Part model, mm, in its own coordinate system. A direction names the side the tool comes from. Round coordinates to 2 decimals unless told otherwise and drop trailing zeros. Write each loop counter-clockwise with the first axis right and the second up, starting at its lowest first coordinate (ties: lowest second). Pieces come first, ordered by that corner, then holes. Notation, with made-up numbers: M 31.5,26.5 L 45.5,26.5 A19 cw 45.5,37.5 Z; hole C 14,27.5 d11. An arc over 180 degrees is marked long. Use a Markdown table: item, result. Add a question column.
1) Slice it at A-A on y = 125. Write the cut outline in (x, z).
2) Wall check: probe 1 along Z at (x, y) = (10.25, 10); probe 2 along Y at (x, z) = (3.9, -100); probe 3 along Y at (x, z) = (40.5, -63). Give the ranges that are in metal, low to high.
3) Slice it at D-D on y = 84.5. Write the cut outline in (x, z).
4) Slice it at C-C on x = 28. Write the cut outline in (y, z), plus the area to 3 significant figures.
5) Two-plate mould, pull along Y, no slides. Class faces 1 (the face through (20, 235, -79)), 2 (the face through (10, 10, -85)), 3 (the face through (10, 0, -79)): released by +Y, released by -Y, zero draft, split by the parting line, or undercut.
6) Which spindle directions (+Z, -Z, +X, -X, +Y, -Y) get a long thin tool onto all of the face, cutting with end or side? Do faces 4 (the face through (2.465, 74.298, -73.629)), 5 (the face through (10, 237, -161)), 6 (the face through (20, 121, -131)). Say none if no direction does.
7) Drop flat-ended pins along their axis: P1, Ø8, axis at y = 102.5, z = -77, coming from the +X side; P2, Ø3, axis at x = 25, y = 46, coming from the -Z side; P3, Ø10, axis at x = 9, y = 14.5, coming from the -Z side. Give the stop position or say it passes through.
8) Slice it at B-B on z = -100. Write the cut outline in (x, y).
```python
from build123d import *

# Parameters (mm, degrees)
EXTRUDE_1_DEPTH          = 200
SKETCH_2_W               = 39
SKETCH_2_H               = 25
CUT_EXTRUDE_1_DEPTH      = 20
SKETCH_3_W               = 126
SKETCH_3_H               = 160
CUT_EXTRUDE_2_DEPTH      = 180
CUT_EXTRUDE_3_REACH      = 362.633
SKETCH_4_R               = 51
SKETCH_5_R               = 25.5
CUT_EXTRUDE_4_DEPTH      = 15
SKETCH_6_R               = 57.15
CUT_EXTRUDE_5_DEPTH      = 5
CUT_EXTRUDE_6_REACH      = 353.875
SKETCH_7_R               = 4.5
PATTERN_CIRCULAR_1_COUNT = 4


with BuildPart() as part:
    # 草图1 → 凸台-拉伸1 (new body)
    with BuildSketch(Plane.XY):
        Polygon((20, 225), (20, 250), (0, 250), (0, 0), (20, 0), (20, 25), (166, 25), (166, 225), align=None)
    extrude(amount=-EXTRUDE_1_DEPTH)

    # 草图2 → 切除-拉伸1 (cut)
    with BuildSketch(Plane.ZY):
        with Locations((-180.5, 237.5)):
            Rectangle(SKETCH_2_W, SKETCH_2_H)
        with Locations((-180.5, 12.5)):
            Rectangle(SKETCH_2_W, SKETCH_2_H)
    extrude(amount=-CUT_EXTRUDE_1_DEPTH, mode=Mode.SUBTRACT)

    # 草图3 → 切除-拉伸2 (cut)
    with BuildSketch(Plane(origin=(0, 0, -200), x_dir=(-1, 0, 0), z_dir=(0, 0, -1))):
        with Locations((-83, 122.583335177)):
            Rectangle(SKETCH_3_W, SKETCH_3_H)
    extrude(amount=-CUT_EXTRUDE_2_DEPTH, mode=Mode.SUBTRACT)

    # 草图4 → 切除-拉伸3 (cut, up to next)
    with BuildSketch(Plane(origin=(166, 0, 0), x_dir=(0, 0, -1), z_dir=(1, 0, 0)), mode=Mode.PRIVATE) as cut_extrude_3_sk1:
        with Locations((100, 125)):
            Circle(SKETCH_4_R)
    cut_extrude_3_tool1 = extrude(cut_extrude_3_sk1.sketch, amount=-CUT_EXTRUDE_3_REACH, mode=Mode.PRIVATE) & part.part
    add(cut_extrude_3_tool1.solids().sort_by_distance((166, 125, -100))[0], mode=Mode.SUBTRACT)

    # 草图5 → 切除-拉伸4 (cut)
    with BuildSketch(Plane(origin=(20, 0, 0), x_dir=(0, 0, -1), z_dir=(1, 0, 0))):
        with Locations(Location((100, 125, 0), (0, 0, 90))):
            Circle(SKETCH_5_R)
    extrude(amount=-CUT_EXTRUDE_4_DEPTH, mode=Mode.SUBTRACT)

    # 草图6 → 切除-拉伸5 (cut)
    with BuildSketch(Plane.ZY):
        with Locations((-100, 125)):
            Circle(SKETCH_6_R)
    extrude(amount=-CUT_EXTRUDE_5_DEPTH, mode=Mode.SUBTRACT)

    # 草图7 → 切除-拉伸6 (cut, up to next)
    with BuildSketch(Plane(origin=(20, 0, 0), x_dir=(0, 0, -1), z_dir=(1, 0, 0)), mode=Mode.PRIVATE) as cut_extrude_6_sk1:
        with Locations(Location((20, 240, 0), (0, 0, 90))):
            Circle(SKETCH_7_R)
    cut_extrude_6_tool1 = extrude(cut_extrude_6_sk1.sketch, amount=-CUT_EXTRUDE_6_REACH, mode=Mode.PRIVATE) & part.part
    # 草图7 → 切除-拉伸6 (cut, up to next)
    with BuildSketch(Plane(origin=(20, 0, 0), x_dir=(0, 0, -1), z_dir=(1, 0, 0)), mode=Mode.PRIVATE) as cut_extrude_6_sk2:
        with Locations(Location((80.5, 240, 0), (0, 0, 90))):
            Circle(SKETCH_7_R)
    cut_extrude_6_tool2 = extrude(cut_extrude_6_sk2.sketch, amount=-CUT_EXTRUDE_6_REACH, mode=Mode.PRIVATE) & part.part
    # 草图7 → 切除-拉伸6 (cut, up to next)
    with BuildSketch(Plane(origin=(20, 0, 0), x_dir=(0, 0, -1), z_dir=(1, 0, 0)), mode=Mode.PRIVATE) as cut_extrude_6_sk3:
        with Locations(Location((141, 240, 0), (0, 0, 90))):
            Circle(SKETCH_7_R)
    cut_extrude_6_tool3 = extrude(cut_extrude_6_sk3.sketch, amount=-CUT_EXTRUDE_6_REACH, mode=Mode.PRIVATE) & part.part
    # 草图7 → 切除-拉伸6 (cut, up to next)
    with BuildSketch(Plane(origin=(20, 0, 0), x_dir=(0, 0, -1), z_dir=(1, 0, 0)), mode=Mode.PRIVATE) as cut_extrude_6_sk4:
        with Locations(Location((141, 10, 0), (0, 0, 180))):
            Circle(SKETCH_7_R)
    cut_extrude_6_tool4 = extrude(cut_extrude_6_sk4.sketch, amount=-CUT_EXTRUDE_6_REACH, mode=Mode.PRIVATE) & part.part
    # 草图7 → 切除-拉伸6 (cut, up to next)
    with BuildSketch(Plane(origin=(20, 0, 0), x_dir=(0, 0, -1), z_dir=(1, 0, 0)), mode=Mode.PRIVATE) as cut_extrude_6_sk5:
        with Locations(Location((80.5, 10, 0), (0, 0, 180))):
            Circle(SKETCH_7_R)
    cut_extrude_6_tool5 = extrude(cut_extrude_6_sk5.sketch, amount=-CUT_EXTRUDE_6_REACH, mode=Mode.PRIVATE) & part.part
    # 草图7 → 切除-拉伸6 (cut, up to next)
    with BuildSketch(Plane(origin=(20, 0, 0), x_dir=(0, 0, -1), z_dir=(1, 0, 0)), mode=Mode.PRIVATE) as cut_extrude_6_sk6:
        with Locations(Location((20, 10, 0), (0, 0, 180))):
            Circle(SKETCH_7_R)
    cut_extrude_6_tool6 = extrude(cut_extrude_6_sk6.sketch, amount=-CUT_EXTRUDE_6_REACH, mode=Mode.PRIVATE) & part.part
    add(cut_extrude_6_tool1.solids().sort_by_distance((20, 240, -20))[0], mode=Mode.SUBTRACT)
    add(cut_extrude_6_tool2.solids().sort_by_distance((20, 240, -80.5))[0], mode=Mode.SUBTRACT)
    add(cut_extrude_6_tool3.solids().sort_by_distance((20, 240, -141))[0], mode=Mode.SUBTRACT)
    add(cut_extrude_6_tool4.solids().sort_by_distance((20, 10, -141))[0], mode=Mode.SUBTRACT)
    add(cut_extrude_6_tool5.solids().sort_by_distance((20, 10, -80.5))[0], mode=Mode.SUBTRACT)
    add(cut_extrude_6_tool6.solids().sort_by_distance((20, 10, -20))[0], mode=Mode.SUBTRACT)

    # 草图9 → M12 螺纹孔1 (revolve, cut)
    with BuildSketch(Plane(origin=(166, 195.711356231, -170.71), x_dir=(0, 0, -1), z_dir=(0, 1, 0))):
        Polygon((0, 0), (0, 29.25), (5.1, 26.185610843), (5.1, 0), align=None)
    hole_wizard_m12_1 = revolve(axis=Axis((172.35, 195.711356231, -170.71), (-1, 0, 0)), mode=Mode.SUBTRACT)

    # 阵列(圆周)1: M12 螺纹孔1 ×4 about axis
    pattern_circular_1_axis = Axis((0, 125, -100), (1, 0, 0))
    for i in range(1, PATTERN_CIRCULAR_1_COUNT):
        add(hole_wizard_m12_1.rotate(pattern_circular_1_axis, i * 360 / PATTERN_CIRCULAR_1_COUNT), mode=Mode.SUBTRACT)


solid = part.part
```
Entries:
| question | item | result |
|---|---|---|
| 1 | outline | M 0,-200 L 20,-200 L 20,-125.5 L 5,-125.5 L 5,-157.15 L 0,-157.15 Z; M 0,-42.85 L 5,-42.85 L 5,-74.5 L 20,-74.5 L 20,-20 L 146,-20 L 146,-49 L 166,-49 L 166,0 L 0,0 Z; M 146,-200 L 166,-200 L 166,-151 L 146,-151 Z |
| 2 | probe 1 | z = -161 to -145.5, -136.5 to -85, -76 to -24.5, -15.5 to 0 |
| 2 | probe 2 | y = 0 to 67.85, 182.15 to 250 |
| 2 | probe 3 | y = 25 to 42.58, 202.58 to 225 |
| 3 | outline | M 0,-200 L 20,-200 L 20,-20 L 146,-20 L 146,-69 L 166,-69 L 166,0 L 0,0 L 0,-59.68 L 5,-59.68 L 5,-140.32 L 0,-140.32 Z; M 146,-200 L 166,-200 L 166,-131 L 146,-131 Z |
| 4 | outline | M 25,-200 L 42.58,-200 L 42.58,-20 L 202.58,-20 L 202.58,-200 L 225,-200 L 225,0 L 25,0 Z |
| 4 | area | 11,200 mm^2 |
| 5 | face 1 | zero draft |
| 5 | face 2 | undercut |
| 5 | face 3 | released by -Y |
| 6 | face 4 | -X |
| 6 | face 5 | -Z, +X, -X, +Y |
| 6 | face 6 | -Z |
| 7 | P1 | stops at x = 20 |
| 7 | P2 | stops at z = -20 |
| 7 | P3 | stops at z = -161 |
| 8 | outline | M 0,0 L 20,0 L 20,25 L 166,25 L 166,74 L 146,74 L 146,42.58 L 20,42.58 L 20,99.5 L 5,99.5 L 5,67.85 L 0,67.85 Z; M 0,182.15 L 5,182.15 L 5,150.5 L 20,150.5 L 20,202.58 L 146,202.58 L 146,176 L 166,176 L 166,225 L 20,225 L 20,250 L 0,250 Z |
